Read the model definition and answer for the solid it produces. Units are mm, in the model's axes. Face numbers are marked on the shaded views. A direction names the side the tool comes from. Coordinates: 2 decimals unless noted, no trailing zeros. Write each loop counter-clockwise with the first axis right and the second up, starting at its lowest first coordinate (ties: lowest second). Pieces come first, ordered by that corner, then holes. Notation, with made-up numbers: (87, 38) -> (112, 38) arc R30 cw to (112, 71) -> close; hole circle Ø8 at (5, 72). An arc over 180 degrees is marked (long way). Answer as a JSON object with one key per item and string values. Group by question number.
(1) Find section C-C (y = 506.5). Give the vertices of the cut face in (x, z), then the cut area to 3 significant figures.
(2) Find section B-B (x = 698.75). Give the vertices of the cut face in (y, z).
(3) A flat-ended cylindrical pin translates along its axis: P1, Ø1, axis at x = 712.5, z = 2, coming from the +Y side. Find the tip coordinate at first contact, or state that the pin passes through.
(4) Find section A-A (z = 0.55). Give the vertices of the cut face in (x, y), then the cut area to 3 significant figures.
(5) Which of the six approach directions +Z, -Z, +X, -X, +Y, -Y give full straight-line access (tool end or side, diameter ignored) to the marked faces 4 and 5?
(6) For a pull along X with two mould halves and no side action, classify the marked faces 1, 2 and 3 as +X half, -X half, draft (parallel to the pull), parting line (faces both ways), or undercut.
(7) Straight lines are drawn through the part: L1, parallel to Y at x = 703, z = 1.1; L2, parallel to Y at x = 702, z = 0.25; L3, parallel to X at y = 503, z = 1.05. For each, find the intervals that lie inside material, in ascending order.
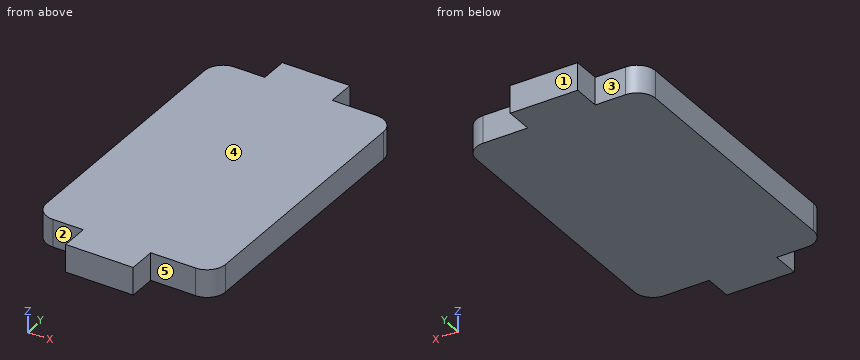
from build123d import *

# Parameters (mm, degrees)
BASE_EXTRUDE_DEPTH = 3


with BuildPart() as part:
    # Sketch1 → Base-Extrude (new body)
    with BuildSketch(Plane.XY):
        with BuildLine():
            Line((701.562436995, 484.642265501), (701.672859679, 487.640232618))
            Line((701.672859679, 487.640232618), (698.38928136, 487.761175083))
            ThreePointArc((698.38928136, 487.761175083), (696.997587478, 488.398618328), (696.464251738, 489.83343495))
            Line((696.464251738, 489.83343495), (697.458055899, 516.815138997))
            ThreePointArc((697.458055899, 516.815138997), (698.095499144, 518.206832879), (699.530315766, 518.740168618))
            Line((699.530315766, 518.740168618), (702.813894085, 518.619226153))
            Line((702.813894085, 518.619226153), (702.92431677, 521.61719327))
            Line((702.92431677, 521.61719327), (710.26431677, 521.346842571))
            Line((710.26431677, 521.346842571), (710.153894085, 518.348875455))
            Line((710.153894085, 518.348875455), (715.015630112, 518.169805464))
            ThreePointArc((715.015630112, 518.169805464), (716.407323993, 517.532362219), (716.940659733, 516.097545597))
            Line((716.940659733, 516.097545597), (715.946855573, 489.11584155))
            ThreePointArc((715.946855573, 489.11584155), (715.309412328, 487.724147668), (713.874595706, 487.190811929))
            Line((713.874595706, 487.190811929), (709.012859679, 487.369881919))
            Line((709.012859679, 487.369881919), (708.902436995, 484.371914803))
            Line((708.902436995, 484.371914803), (701.562436995, 484.642265501))
        make_face()
    extrude(amount=BASE_EXTRUDE_DEPTH)


solid = part.part
Results below:
{
 "1": {"outline": "(697.08, 0) -> (716.59, 0) -> (716.59, 3) -> (697.08, 3) -> close", "area": "58.5 mm2"},
 "2": {"outline": "(487.75, 0) -> (518.61, 0) -> (518.61, 3) -> (487.75, 3) -> close"},
 "3": {"P1": "stops at y = 518.28"},
 "4": {"outline": "(696.46, 489.83) arc R2 ccw to (698.39, 487.76) -> (701.67, 487.64) -> (701.56, 484.64) -> (708.9, 484.37) -> (709.01, 487.37) -> (713.87, 487.19) arc R2 ccw to (715.95, 489.12) -> (716.94, 516.1) arc R2 ccw to (715.02, 518.17) -> (710.15, 518.35) -> (710.26, 521.35) -> (702.92, 521.62) -> (702.81, 518.62) -> (699.53, 518.74) arc R2 ccw to (697.46, 516.82) -> close", "area": "645 mm2"},
 "5": {"face 4": "+Z, +X, -X, +Y, -Y", "face 5": "+Z, -Z, -Y"},
 "6": {"face 1": "+X half", "face 2": "-X half", "face 3": "undercut"},
 "7": {"L1": "y = 484.59 to 521.61", "L2": "y = 484.63 to 518.65", "L3": "x = 696.95 to 716.46"}
}
